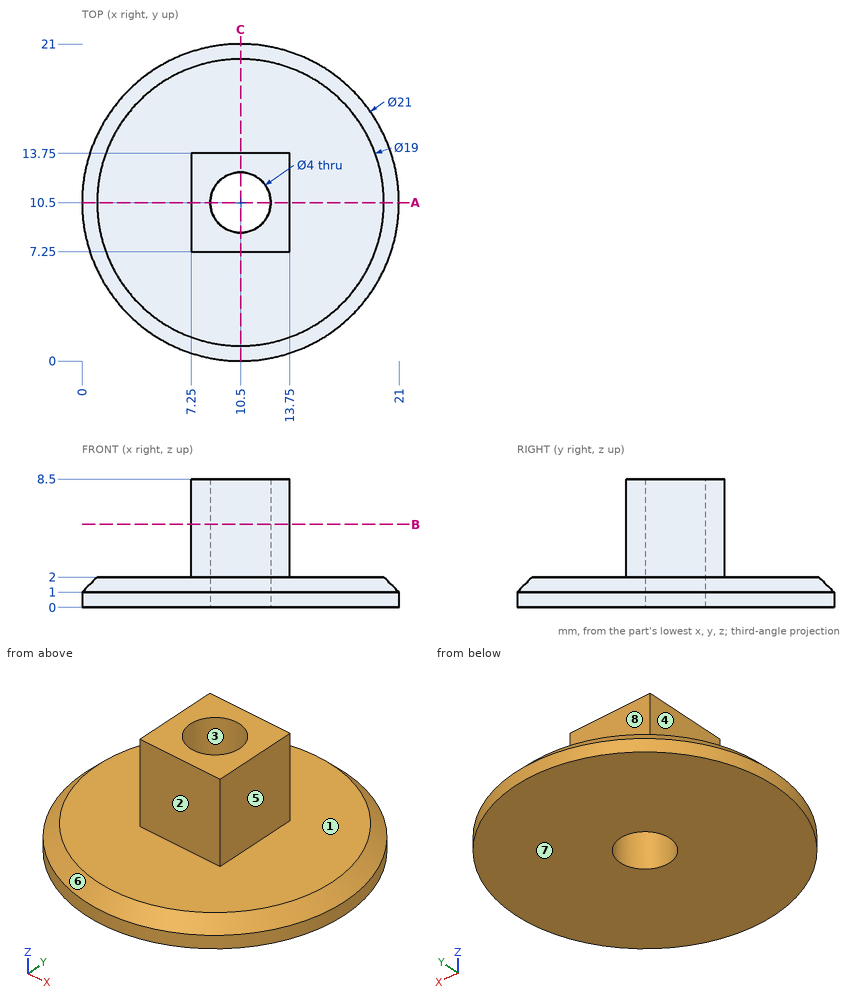
Here's the drawing with two shaded views (mm, measured from the low corner). I have some questions. A direction names the side the tool comes from. Coordinates: 2 decimals unless noted, no trailing zeros. Loops run counter-clockwise (first coordinate to the right, second up) from the corner with the lowest first, then second, coordinate; pieces in that order, holes last. Notation, with made-up numbers: (-33.5, -17) -> (-10.5, -17) arc R33 ccw to (-10.5, 22) -> close; hole circle Ø3 at (17.25, -26.5). An arc over 180 degrees is marked (long way). Put each result on its own line as item: value. Start each with the question number.
Q1. Thinking about a two-plate mould opening in Y: for the marked faces 1, 2 and 3, which applies, pulls with the +Y half, pulls with the -Y half, needs draft (parallel to the pull), parting line crosses it, or undercut?
Q2. I want a section at B-B (z = 5.5). Write out the boundary of the cut face in (x, y), plus the area to 3 significant figures.
Q3. If I drill on line 1 (X direction, y = 10.5, z = 3.75); line 2 (Z direction, x = 12.5, y = 5), over which ranges is the centre line in solid material (lowest first)? Write a range as [from, to].
Q4. For the marked faces 4, 5, 6, 7 and 8, which set-ups out of +Z, -Z, +X, -X, +Y, -Y let a thin tool reach every point of the face, with its end or its side?
Q5. I'm going to push flat-ended pins straight in: P1, Ø1.5, axis at x = 9.5, y = 16, coming from the -Z side; P2, Ø5, axis at y = 11, z = 4, coming from the +X side; P3, Ø12, axis at x = 18, y = 2.5, coming from the +Z side; P4, Ø2, axis at x = 9, z = 6, coming from the +Y side. Where does each tip first touch, or does it pass through?
Q6. I want a section at A-A (y = 10.5). Write out the boundary of the cut face in (x, z), plus the area to 4 significant figures.
Taken from the geometry:
1. face 1: needs draft
1. face 2: pulls with the -Y half
1. face 3: undercut
2. outline: (7.25, 7.25) -> (13.75, 7.25) -> (13.75, 13.75) -> (7.25, 13.75) -> close; hole circle Ø4 at (10.5, 10.5)
2. area: 29.7 mm2
3. line 1: x = [7.25, 8.5], [12.5, 13.75]
3. line 2: z = [0, 2]
4. face 4: +Z, -X, +Y, -Y
4. face 5: +Z, +X, +Y, -Y
4. face 6: +Z
4. face 7: -Z, +X, -X, +Y, -Y
4. face 8: +Z, +X, -X, +Y
5. P1: stops at z = 0
5. P2: stops at x = 20.49
5. P3: stops at z = 2
5. P4: stops at y = 13.75
6. outline: (0, 0) -> (8.5, 0) -> (8.5, 8.5) -> (7.25, 8.5) -> (7.25, 2) -> (1, 2) -> (0, 1) -> close; (12.5, 0) -> (21, 0) -> (21, 1) -> (20, 2) -> (13.75, 2) -> (13.75, 8.5) -> (12.5, 8.5) -> close
6. area: 49.25 mm2
